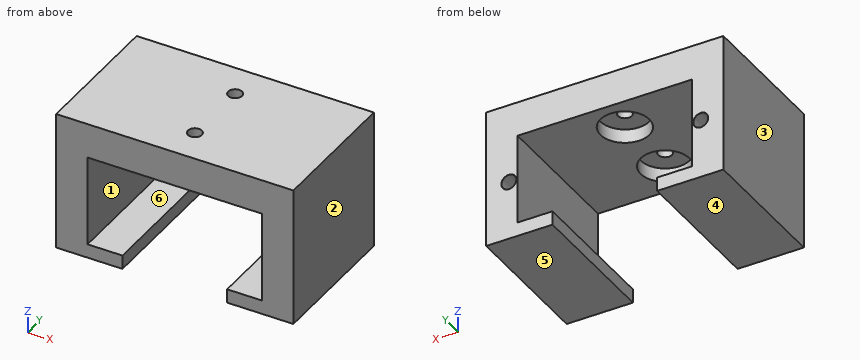
Autodesk Inventor part; units mm, degrees
ref_plane "YZ Plane" through (0, 0, 0) normal (1, 0, 0) x (0, 1, 0)
ref_plane "XZ Plane" through (0, 0, 0) normal (0, 1, 0) x (-1, 0, 0)
ref_plane "XY Plane" through (0, 0, 0) normal (0, 0, 1) x (1, 0, 0)
sketch "Sketch1" plane through (0, 0, 0) normal (0, 1, 0) x (-1, 0, 0)
  line L0 (0, 0) -> (34, 0)
  line L1 (34, 0) -> (34, -20)
  line L2 (34, -20) -> (0, -20)
  line L3 (0, -20) -> (0, 0)
  dimension "d0" = 34
  dimension "d1" = 20
extrude "Extrusion1" add sketch "Sketch1" along normal blind 20
sketch "Sketch2" plane through (0, 20, 0) normal (0, 1, 0) x (1, 0, 0)
  line L0 (-29.5, 18) -> (-4.5, 18)
  line L1 (-4.5, 18) -> (-4.5, 5)
  line L2 (-4.5, 5) -> (-29.5, 5)
  line L3 (-29.5, 5) -> (-29.5, 18)
  line L4 (0, 20) -> (-34, 20)
  line L5 (-34, 20) -> (-34, 0)
  line L6 (-24.5, 20) -> (-9.5, 20)
  line L7 (-9.5, 20) -> (-9.5, 18)
  line L8 (-9.5, 18) -> (-24.5, 18)
  line L9 (-24.5, 18) -> (-24.5, 20)
  line L10 (0, 0) -> (0, 20)
  point P0 (-9.5, 20)
  dimension "d6" = 25
  dimension "d7" = 13
  dimension "d8" = 2
  dimension "d9" = 4.5
  dimension "d12" = 5
  dimension "d13" = 5
  dimension "d26" = 4.5
extrude "Extrusion2" cut sketch "Sketch2" against normal blind 33
sketch "Sketch3" plane through (-4.5, 20, -5) normal (0, 0, -1) x (-1, 0, 0)
  line L0 (29.5, -20) -> (29.5, 0)
  line L1 (-4.5, -20) -> (-4.5, 0)
  line L2 (29.5, 0) -> (-4.5, 0)
  line L3 (12.5, 0) -> (12.5, -20)
  circle A0 centre (12.5, -5) radius 1
  circle A1 centre (12.5, -15) radius 1
  dimension "d27" = 2
  dimension "d28" = 2
  dimension "d29" = 5
  dimension "d30" = 5
  dimension "d33" = 10
extrude "Extrusion3" cut sketch "Sketch3" against normal through all
sketch "Sketch4" plane through (0, 20, 0) normal (0, 1, 0) x (1, 0, 0)
  line L0 (-34, 20) -> (-34, 0)
  line L1 (-29.5, 18) -> (-29.5, 5)
  line L2 (-9.5, 18) -> (-4.5, 18)
  line L3 (-29.5, 5) -> (-4.5, 5)
  line L4 (-4.5, 5) -> (-4.5, 18)
  line L5 (-4.5, 18) -> (-29.5, 18)
  line L6 (-29.5, 18) -> (-29.5, 5)
  line L7 (-29.5, 11.5) -> (-34, 11.5)
  line L8 (-29.5, 11.5) -> (0, 11.5)
  line L9 (0, 0) -> (0, 20)
  circle A0 centre (-3.25, 11.5) radius 0.8
  circle A1 centre (-30.75, 11.5) radius 0.8
  dimension "d21" = 1.6
  dimension "d22" = 3.25
  dimension "d31" = 1.6
  dimension "d32" = 3.25
hole "Hole1" at (-30.75, 20, -11.5) at (-3.25, 20, -11.5) direction (0, -1, 0) diameter 2.1211 depth 7.1 tip angle 118 countersink diameter 2.159 countersink angle 82
sketch "Sketch6" plane through (-4.5, 20, -5) normal (0, 0, -1) x (-1, 0, 0)
  line L0 (29.5, -20) -> (29.5, 0)
  line L1 (-4.5, -20) -> (-4.5, 0)
  line L2 (29.5, 0) -> (-4.5, 0)
  line L3 (12.5, 0) -> (12.5, -20)
  circle A0 centre (12.5, -5) radius 1
  circle A1 centre (12.5, -15) radius 1
  circle A2 centre (12.5, -5) radius 1
  circle A3 centre (12.5, -5) radius 3.5
  circle A4 centre (12.5, -15) radius 3.5
  dimension "d41" = 2
  dimension "d42" = 2
  dimension "d43" = 5
  dimension "d44" = 5
  dimension "d45" = 10
  dimension "d46" = 7
  dimension "d47" = 7
extrude "Extrusion5" cut sketch "Sketch6" against normal blind 2 contours A3 L3 A0 | A4 L3 A1 | L3 A1 A4 | L3 A0 A3
properties part number "Servo Holder"
Work out the finished part from the listing and answer in its coordinate system (mm). Face numbers are marked on the shaded views. A direction names the side the tool comes from. Coordinates: 2 decimals unless noted, no trailing zeros. Loops run counter-clockwise (first coordinate to the right, second up) from the corner with the lowest first, then second, coordinate; pieces in that order, holes last. Notation, with made-up numbers: M 42,35 L 83,35 A21 cw 83,68 Z; hole C 62.25,50 d6. An arc over 180 degrees is marked long. Answer in a Markdown table with one row per item. Add a question column.
1. Consider L1, parallel to Y at x = -17, z = -3.9; L2, parallel to Y at x = -17, z = -2.4; L3, parallel to Z at x = -30.75, y = 17.75. Determine where each line is inside the solid, lowest interval first.
2. Find section B-B, the plane z = -5.5. Write down the section's boundary in (x, y), then the cut area to 3 significant figures.
3. Find section C-C, the plane x = -26. Write down the section's boundary in (y, z), then the cut area to 3 significant figures.
4. Flat-ended cylindrical pins translate along their axes: P1, Ø6, axis at x = -20, y = 14, coming from the +Z side; P2, Ø7.5, axis at x = -18, y = 6, coming from the -Z side; P3, Ø2.5, axis at x = -17, y = 5, coming from the -Z side. Find the tip coordinate at first contact, or state that the pin passes through.
5. Find section A-A, the plane x = -17. Write down the section's boundary in (y, z).
6. A tool of negligible diameter and unlimited length cuts with its end or side. For the marked faces 5 and 6, from which of +Z, -Z, +X, -X, +Y, -Y can it reach the whole face along a straight path? Write none if from no direction.
7. The mould has two halves that part along X. Classify the marked faces 1, 2, 3 and 4: pulls with the +X half, pulls with the -X half, needs draft (parallel to the pull), parting line crosses it, or undercut.
8. Find section D-D, the plane y = 5. Write down the section's boundary in (x, z).
Reported:
| question | item | result |
|---|---|---|
| 1 | L1 | y = 0 to 1.5, 8.5 to 11.5, 18.5 to 20 |
| 1 | L2 | y = 0 to 4, 6 to 14, 16 to 20 |
| 1 | L3 | z = -20 to -12.56, -10.44 to 0 |
| 2 | outline | M -34,0 L -29.5,0 L -29.5,20 L -34,20 Z; M -4.5,0 L 0,0 L 0,20 L -4.5,20 Z |
| 2 | area | 180 mm^2 |
| 3 | outline | M 0,-20 L 20,-20 L 20,-18 L 0,-18 Z; M 0,-5 L 20,-5 L 20,0 L 0,0 Z |
| 3 | area | 140 mm^2 |
| 4 | P1 | stops at z = 0 |
| 4 | P2 | stops at z = -5 |
| 4 | P3 | stops at z = -3 |
| 5 | outline | M 0,-5 L 1.5,-5 L 1.5,-3 L 4,-3 L 4,0 L 0,0 Z; M 6,-3 L 8.5,-3 L 8.5,-5 L 11.5,-5 L 11.5,-3 L 14,-3 L 14,0 L 6,0 Z; M 16,-3 L 18.5,-3 L 18.5,-5 L 20,-5 L 20,0 L 16,0 Z |
| 6 | face 5 | -Z, +X, -X, +Y, -Y |
| 6 | face 6 | +Y, -Y |
| 7 | face 1 | undercut |
| 7 | face 2 | pulls with the +X half |
| 7 | face 3 | pulls with the -X half |
| 7 | face 4 | needs draft |
| 8 | outline | M -34,-20 L -24.5,-20 L -24.5,-18 L -29.5,-18 L -29.5,-5 L -20.5,-5 L -20.5,-3 L -18,-3 L -18,0 L -34,0 Z; M -16,-3 L -13.5,-3 L -13.5,-5 L -4.5,-5 L -4.5,-18 L -9.5,-18 L -9.5,-20 L 0,-20 L 0,0 L -16,0 Z |
